Input: dimensioned drawing with shaded views. Units: mm. Origin: part minimum x, y, z. A direction names the side the tool comes from. Give positions to 0.01 mm unless a question says otherwise; leave off trailing zeros. Write each loop counter-clockwise with the first axis right and the second up, starting at its lowest first coordinate (ties: lowest second). Pieces come first, ordered by that corner, then holes. Notation, with made-up numbers: (37.25, -14.75) -> (44.25, -14.75) arc R15 ccw to (44.25, 9.25) -> close; hole circle Ø11 at (-22, -3.5). An arc over 180 degrees is marked (long way). Answer as a JSON object with one key per item and string values. Group by question number.
(1) Material intervals for probe 1 along X at (y, z) = (25.4, 21.25) (3 decimals); probe 2 along Y at (x, z) = (50.8, 21) (3 decimals); probe 3 along X at (y, z) = (42, 32.5), sorted ascending.
(2) Draft query along Z for the marked faces 4, 5 and 6. Return one class per face: +Z half, -Z half, draft (parallel to the pull), parting line (faces both ways), or undercut.
(3) Section query A-A on x = 50.8. Output: boundary loops of the cut face in (y, z) (3 decimals).
(4) Set-up query: the marked faces 1, 2 and 3. Return all of +Z, -Z, +X, -X, +Y, -Y with unobstructed straight access to the full face (end or side cutting, diameter ignored); none if empty.
(5) Section query D-D on y = 15. Output: boundary loops of the cut face in (x, z).
(6) Contact query for flat-ended pins moving along their axis: pin 1 Ø6 at (x, z) = (84.5, 43.5) entering from -Y; pin 2 Ø6 at (x, y) = (104, 7) entering from +Z; pin 3 Ø3 at (y, z) = (21.5, 9) entering from -X; pin 4 Ø15 at (x, y) = (64.5, 18.5) entering from -Z. Output: stop coordinate, or through.
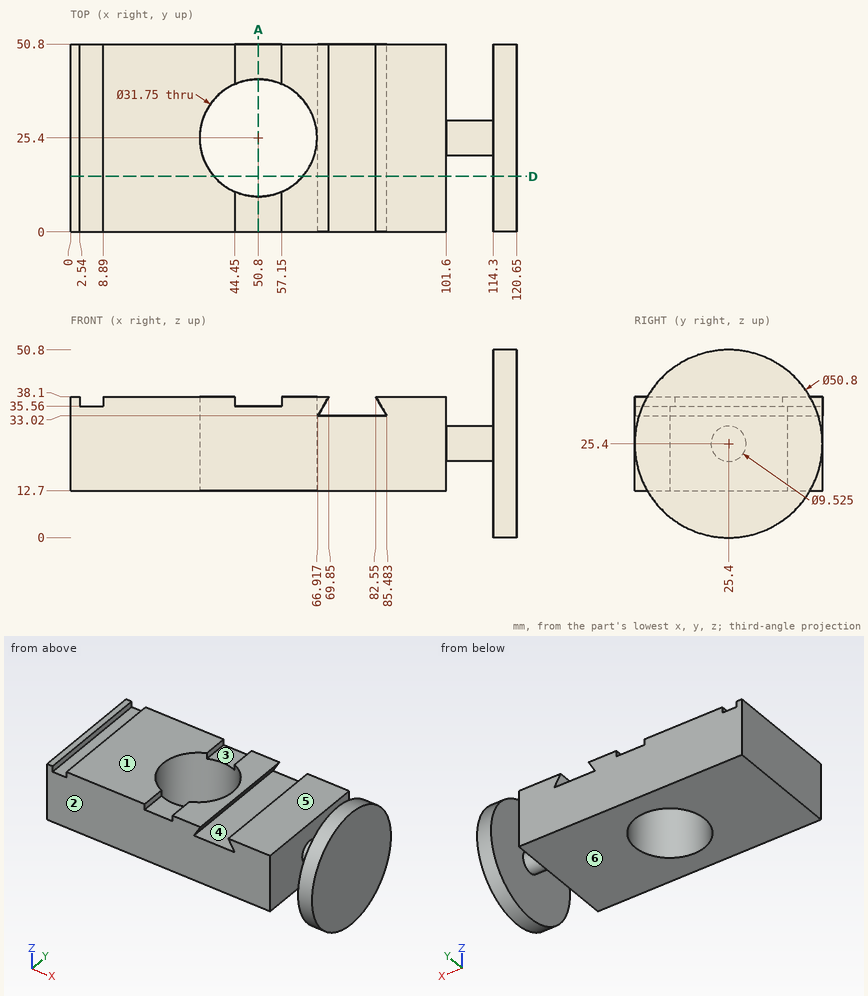
Answer list:
{
 "1": {"probe 1": "0 to 34.925, 66.675 to 120.65", "probe 2": "0 to 9.525, 41.275 to 50.8", "probe 3": "0 to 101.6, 114.3 to 120.65"},
 "2": {"face 4": "undercut", "face 5": "+Z half", "face 6": "-Z half"},
 "3": {"outline": "(0, 12.7) -> (9.525, 12.7) -> (9.525, 35.56) -> (0, 35.56) -> close; (41.275, 12.7) -> (50.8, 12.7) -> (50.8, 35.56) -> (41.275, 35.56) -> close"},
 "4": {"face 1": "+Z, -X, +Y, -Y", "face 2": "+Z, -Z, +X, -X, -Y", "face 3": "+Z, +Y, -Y"},
 "5": {"outline": "(0, 12.7) -> (38.81, 12.7) -> (38.81, 38.1) -> (8.89, 38.1) -> (8.89, 35.56) -> (2.54, 35.56) -> (2.54, 38.1) -> (0, 38.1) -> close; (62.79, 12.7) -> (101.6, 12.7) -> (101.6, 38.1) -> (82.55, 38.1) -> (85.48, 33.02) -> (66.92, 33.02) -> (69.85, 38.1) -> (62.79, 38.1) -> close; (114.3, 2.23) -> (120.65, 2.23) -> (120.65, 48.57) -> (114.3, 48.57) -> close"},
 "6": {"pin 1": "through", "pin 2": "z = 38.1", "pin 3": "x = 114.3", "pin 4": "z = 12.7"}
}
